Part model, mm, in its own coordinate system. A direction names the side the tool comes from. Round coordinates to 2 decimals unless told otherwise and drop trailing zeros. Loops run counter-clockwise (first coordinate to the right, second up) from the corner with the lowest first, then second, coordinate; pieces in that order, holes last. Notation, with made-up numbers: (14, 54) -> (53, 54) arc R5 cw to (53, 60) -> close; hole circle Ø8 at (-31.75, 50.25). An arc over 180 degrees is marked (long way). Use a Markdown table: item, result. Add a question column.
Item 1: Flat gauge pins, fed straight in: pin 1 (6.5 mm diameter, centred on x = 49.5, y = 0.5, fed in from +Z); pin 2 (5 mm diameter, centred on y = -10.5, z = 8.5, fed in from +X); pin 3 (5 mm diameter, centred on x = 20, z = 5.5, fed in from +Y); pin 4 (3.5 mm diameter, centred on x = 56, y = 0, fed in from -Z). Where does each tip first touch, or does it go through?
Item 2: Cut at D-D, the plane z = 2.25. List the corners of the cut face in (x, y), plus the area to 3 significant figures.
Item 3: Probe line 1 (Y direction, x = 26.5, z = 9); line 2 (Y direction, x = 26.5, z = 4.75); line 3 (X direction, y = -8.5, z = 5.25). List the from-to ranges inside material, lowest first. Write a range as [from, to].
Item 4: Which spindle directions (+Z, -Z, +X, -X, +Y, -Y) get a long thin tool onto all of the face, cutting with end or side? Do faces 1 (the face through (-4, -6, 2)), 2 (the face through (33, -11, 7)), 3 (the face through (28, -6.737, 4)). Say none if no direction does.
Item 5: Cut at C-C, the plane x = 0. List the corners of the cut face in (y, z), plus the area to 3 significant figures.
Item 6: Two-plate mould, pull along X, no slides. Class faces 4 (the face through (50.51, -6.216, 1.972)), 5 (the face through (5, -6.4, 4)), 6 (the face through (23, -11, 7)), 7 (the face through (-1.27, -0.97, 1.97)): pulls with the +X half, pulls with the -X half, needs draft (parallel to the pull), parting line crosses it, or undercut.
Item 7: Cut at A-A, the plane z = 9. List the corners of the cut face in (x, y), plus the area to 3 significant figures.
Item 8: Cut at B-B, the plane y = 0. List the corners of the cut face in (x, z), plus the area to 3 significant figures.
```python
from build123d import *

# Parameters (mm, degrees)
CROQUIS1_R              = 1.6
SALIENTE_EXTRUIR1_DEPTH = 4
CROQUIS2_W              = 10
CROQUIS2_H              = 8
SALIENTE_EXTRUIR2_DEPTH = 8
CORTAR_EXTRUIR1_REACH   = 45.564
CROQUIS3_R              = 1.6
REDONDEO1_R             = 2
REDONDEO2_R             = 8
REDONDEO3_R             = 4


with BuildPart() as part:
    # Croquis1 → Saliente-Extruir1 (new body)
    with BuildSketch(Plane.XY):
        with BuildLine():
            Line((-4, -4.737087713), (-4, -14.737087713))
            Line((-4, -14.737087713), (60, -14.737087713))
            Line((60, -14.737087713), (60, -4.737087713))
            ThreePointArc((60, -4.737087713), (56, 6.2), (52, -4.737087713))
            Line((52, -4.737087713), (52, -6.737087713))
            Line((52, -6.737087713), (4, -6.737087713))
            Line((4, -6.737087713), (4, -4.737087713))
            ThreePointArc((4, -4.737087713), (0, 6.2), (-4, -4.737087713))
        make_face()
        Circle(CROQUIS1_R, mode=Mode.SUBTRACT)
        with Locations((56, 0)):
            Circle(CROQUIS1_R, mode=Mode.SUBTRACT)
    extrude(amount=SALIENTE_EXTRUIR1_DEPTH)

    # Croquis2 → Saliente-Extruir2 (add)
    with BuildSketch(Plane.XY.offset(4)):
        with Locations((28, -10.737087713)):
            Rectangle(CROQUIS2_W, CROQUIS2_H)
    extrude(amount=SALIENTE_EXTRUIR2_DEPTH)

    # Croquis3 → Cortar-Extruir1 (cut, up to next)
    with BuildSketch(Plane.ZY.offset(-23), mode=Mode.PRIVATE) as cortar_extruir1_sk1:
        with Locations((9, -10.737087713)):
            Circle(CROQUIS3_R)
    cortar_extruir1_tool1 = extrude(cortar_extruir1_sk1.sketch, amount=-CORTAR_EXTRUIR1_REACH, mode=Mode.PRIVATE) & part.part
    add(cortar_extruir1_tool1.solids().sort_by_distance((23, -10.737088, 9))[0], mode=Mode.SUBTRACT)

    # Redondeo1
    # the kernel refuses this fillet: 2 mm, written as the material it takes off along each edge
    with BuildSketch(Plane(origin=(33, -1.737087713, 12), x_dir=(-1, 0, 0), z_dir=(0, -1, 0))) as redondeo1_piece_1:
        with BuildLine():
            CenterArc((REDONDEO1_R, REDONDEO1_R), REDONDEO1_R, 180, 90)
            Line((0, REDONDEO1_R), (0, 0))
            Line((0, 0), (REDONDEO1_R, 0))
        make_face()
    extrude(amount=18, mode=Mode.SUBTRACT)
    with BuildSketch(Plane(origin=(23, -19.737087713, 12), x_dir=(0, 0, -1), z_dir=(0, 1, 0))) as redondeo1_piece_2:
        with BuildLine():
            CenterArc((REDONDEO1_R, -REDONDEO1_R), REDONDEO1_R, 90, 90)
            Line((0, -REDONDEO1_R), (0, 0))
            Line((0, 0), (REDONDEO1_R, 0))
        make_face()
    extrude(amount=18, mode=Mode.SUBTRACT)
    with BuildSketch(Plane(origin=(18, -6.737087713, 12), x_dir=(0, -1, 0), z_dir=(1, 0, 0))) as redondeo1_piece_3:
        with BuildLine():
            CenterArc((REDONDEO1_R, REDONDEO1_R), REDONDEO1_R, 180, 90)
            Line((0, REDONDEO1_R), (0, 0))
            Line((0, 0), (REDONDEO1_R, 0))
        make_face()
    extrude(amount=20, mode=Mode.SUBTRACT)
    with BuildSketch(Plane(origin=(38, -14.737087713, 12), x_dir=(0, 0, -1), z_dir=(-1, 0, 0))) as redondeo1_piece_4:
        with BuildLine():
            CenterArc((REDONDEO1_R, -REDONDEO1_R), REDONDEO1_R, 90, 90)
            Line((0, -REDONDEO1_R), (0, 0))
            Line((0, 0), (REDONDEO1_R, 0))
        make_face()
    extrude(amount=20, mode=Mode.SUBTRACT)

    # Redondeo2
    redondeo2_edges = [part.edges().sort_by_distance(p)[0] for p in [
        (60, -14.737087713, 2),
        (-4, -14.737087713, 2),
    ]]
    fillet(redondeo2_edges, radius=REDONDEO2_R)

    # Redondeo3
    # the kernel refuses this fillet: 4 mm, written as the material it adds along each edge
    with BuildSketch(Plane(origin=(52, -6.737087713, 0), x_dir=(-1, 0, 0), z_dir=(0, 0, 1))) as redondeo3_piece_1:
        with BuildLine():
            CenterArc((3.464101615, -4), REDONDEO3_R, 90, 60)
            Line((0, -2), (-0.069282032, -1.96))
            ThreePointArc((-0.069282032, -1.96), (-0.08, -1), (-0.08, 0))
            Line((-0.08, 0), (0, 0.08))
            Line((0, 0.08), (3.464101615, 0.08))
            Line((3.464101615, 0.08), (3.464101615, 0))
        make_face()
    extrude(amount=4)
    with BuildSketch(Plane(origin=(4, -6.737087713, 0), x_dir=(0, 1, 0), z_dir=(0, 0, 1))) as redondeo3_piece_2:
        with BuildLine():
            CenterArc((4, -3.464101615), REDONDEO3_R, 120, 60)
            Line((0, -3.464101615), (-0.08, -3.464101615))
            Line((-0.08, -3.464101615), (-0.08, 0))
            Line((-0.08, 0), (0, 0.08))
            ThreePointArc((0, 0.08), (1, 0.08), (1.96, 0.069282032))
            Line((1.96, 0.069282032), (2, 0))
        make_face()
    extrude(amount=4)


solid = part.part
```
A:
| question | item | result |
|---|---|---|
| 1 | pin 1 | stops at z = 4 |
| 1 | pin 2 | stops at x = 33 |
| 1 | pin 3 | stops at y = -6.74 |
| 1 | pin 4 | stops at z = 0 |
| 2 | outline | (-4, -6.74) arc R8 ccw to (4, -14.74) -> (52, -14.74) arc R8 ccw to (60, -6.74) -> (60, -4.74) arc R6.2 ccw (long way) to (52, -4.74) arc R4 cw to (48.54, -6.74) -> (7.46, -6.74) arc R4 cw to (4, -4.74) arc R6.2 ccw (long way) to (-4, -4.74) -> close; hole circle Ø3.2 at (0, 0); hole circle Ø3.2 at (56, 0) |
| 2 | area | 730 mm^2 |
| 3 | line 1 | y = [-14.74, -12.34], [-9.14, -6.74] |
| 3 | line 2 | y = [-14.74, -6.74] |
| 3 | line 3 | x = [23, 33] |
| 4 | face 1 | +Z, -Z, -X, -Y |
| 4 | face 2 | +Z, +X, +Y, -Y |
| 4 | face 3 | +Z, -Z, +Y |
| 5 | outline | (-13.67, 0) -> (-1.6, 0) -> (-1.6, 4) -> (-13.67, 4) -> close; (1.6, 0) -> (6.2, 0) -> (6.2, 4) -> (1.6, 4) -> close |
| 5 | area | 66.7 mm^2 |
| 6 | face 4 | undercut |
| 6 | face 5 | needs draft |
| 6 | face 6 | pulls with the -X half |
| 6 | face 7 | undercut |
| 7 | outline | (23, -14.74) -> (33, -14.74) -> (33, -12.34) -> (23, -12.34) -> close; (23, -9.14) -> (33, -9.14) -> (33, -6.74) -> (23, -6.74) -> close |
| 7 | area | 48.0 mm^2 |
| 8 | outline | (-6.2, 0) -> (-1.6, 0) -> (-1.6, 4) -> (-6.2, 4) -> close; (1.6, 0) -> (6.2, 0) -> (6.2, 4) -> (1.6, 4) -> close; (49.8, 0) -> (54.4, 0) -> (54.4, 4) -> (49.8, 4) -> close; (57.6, 0) -> (62.2, 0) -> (62.2, 4) -> (57.6, 4) -> close |
| 8 | area | 73.6 mm^2 |
